Part model, mm, in its own coordinate system. Round coordinates to 2 decimals unless told otherwise and drop trailing zeros. Loops run counter-clockwise (first coordinate to the right, second up) from the corner with the lowest first, then second, coordinate; pieces in that order, holes last. Notation, with made-up numbers: (-5.75, 55) -> (16.25, 55) arc R7 ccw to (16.25, 62) -> close; hole circle Ø10 at (78.5, 53). An arc over 180 degrees is marked (long way). Answer as CSV lines item,"result".
from build123d import *

# Parameters (mm, degrees)
SKETCH_R     = 9.5
PAD_DEPTH    = 12.7
SKETCH001_R  = 6.35
POCKET_DEPTH = 6.35
CHAMFER_SIZE = 1


with BuildPart() as part:
    # Sketch → Pad (new body)
    with BuildSketch(Plane.XY):
        Circle(SKETCH_R)
    extrude(amount=PAD_DEPTH)

    # Sketch001 (on Face2 of Pad) → Pocket (cut)
    with BuildSketch(Plane(origin=(0, 0, 0), x_dir=(1, 0, 0), z_dir=(0, 0, -1))):
        Circle(SKETCH001_R)
    extrude(amount=-POCKET_DEPTH, mode=Mode.SUBTRACT)

    # Chamfer
    chamfer_edges = [part.edges().sort_by_distance(p)[0] for p in [
        (-6.35, 0, 6.35),
    ]]
    chamfer(chamfer_edges, length=CHAMFER_SIZE)


solid = part.part
Q1. Drop flat-ended pins along their axis: P1, Ø1.5, axis at y = -3.5, z = 7, coming from the +X side; P2, Ø1, axis at y = 7.5, z = 2.5, coming from the +X side; P3, Ø3, axis at x = 0, y = -2, coming from the -Z side; P4, Ø4, axis at y = -1.5, z = 3.5, coming from the +X side. Give the stop position or say it passes through.
Geometry results:
P1,"x = 9.09"
P2,"x = 6.42"
P3,"z = 6.35"
P4,"x = 9.5"
Q2. Saw through at C-C, the plane z = 3. Write the cut outline in (x, y).
Geometry results:
outline,"circle Ø19 at (0, 0); hole circle Ø12.7 at (0, 0)"
Q3. Drill centre lines: line 1 along Y through (x, z) = (0, 4.2); line 2 along Y through (x, z) = (-3, 5); line 3 along Z through (x, y) = (1, 2.75). Where is each one in solid material? Low to high.
Geometry results:
line 1,"-9.5 to -6.35, 6.35 to 9.5"
line 2,"-9.01 to -5.6, 5.6 to 9.01"
line 3,"6.35 to 12.7"
Q4. Saw through at D-D, the plane z = 9.25. Write the cut outline in (x, y).
Geometry results:
outline,"circle Ø19 at (0, 0)"
Q5. Saw through at A-A, the plane x = 0. Write the cut outline in (y, z).
Geometry results:
outline,"(-9.5, 0) -> (-6.35, 0) -> (-6.35, 5.35) -> (-5.35, 6.35) -> (5.35, 6.35) -> (6.35, 5.35) -> (6.35, 0) -> (9.5, 0) -> (9.5, 12.7) -> (-9.5, 12.7) -> close"
Q6. Two-plate mould, pull along X, no slides. Class faces 1 (the face through (0, 0, 12.7)), 2 (the face through (0, 0, 6.35)), 3 (the face through (-1.38, 6.2, 2.64)), 4 (the face through (4.38, -8.43, 6.26)): pulls with the +X half, pulls with the -X half, needs draft (parallel to the pull), parting line crosses it, or undercut.
Geometry results:
face 1,"needs draft"
face 2,"undercut"
face 3,"undercut"
face 4,"parting line crosses it"
